Design review of the part built by this model. Coordinates are the model's own, in mm. A direction names the side the tool comes from. Give positions to 0.01 mm unless a question says otherwise; leave off trailing zeros. Write each loop counter-clockwise with the first axis right and the second up, starting at its lowest first coordinate (ties: lowest second). Pieces come first, ordered by that corner, then holes. Notation, with made-up numbers: M -39,69.25 L -32,69.25 A24 cw -32,85.25 Z; hole C 59,-37 d4. An arc over 180 degrees is marked long. One line per item, written item: value. Start each with the question number.
```python
from build123d import *

# Parameters (mm, degrees)
SKETCH1_W           = 80
SKETCH1_H           = 4
SKETCH1_W_2         = 10
BOSS_EXTRUDE1_DEPTH = 20
CUT_EXTRUDE2_REACH  = 92
SKETCH2_R           = 2.7
CUT_EXTRUDE3_REACH  = 14
SKETCH4_R           = 1.7
SKETCH5_R           = 3.7
SKETCH5_R_2         = 1.7
BOSS_EXTRUDE2_DEPTH = 3
SKETCH6_R           = 4.3
CUT_EXTRUDE4_DEPTH  = 5
CUT_EXTRUDE5_DEPTH  = 3


with BuildPart() as part:
    # Sketch1 → Boss-Extrude1 (new body)
    with BuildSketch(Plane(origin=(0, 0, 0), x_dir=(1, 0, 0), z_dir=(0, 1, 0))):
        with Locations((40, -2)):
            Rectangle(SKETCH1_W, SKETCH1_H)
        Polygon((80, 8), (80, 0), (80, -4), (80, -40.5), (90, -40.5), (90, -36.5), (90, 4), (90, 8), align=None)
        with Locations((95, 6)):
            Rectangle(SKETCH1_W_2, SKETCH1_H)
        with Locations((95, -38.5)):
            Rectangle(SKETCH1_W_2, SKETCH1_H)
    extrude(amount=BOSS_EXTRUDE1_DEPTH)

    # Sketch2 → Cut-Extrude2 (cut, up to next)
    with BuildSketch(Plane(origin=(90, 0, 0), x_dir=(0, 0, -1), z_dir=(1, 0, 0)), mode=Mode.PRIVATE) as cut_extrude2_sk1:
        with Locations((-16.25, 10)):
            Circle(SKETCH2_R)
    cut_extrude2_tool1 = extrude(cut_extrude2_sk1.sketch, amount=-CUT_EXTRUDE2_REACH, mode=Mode.PRIVATE) & part.part
    add(cut_extrude2_tool1.solids().sort_by_distance((90, 10, 16.25))[0], mode=Mode.SUBTRACT)

    # Sketch4 → Cut-Extrude3 (cut, up to next)
    with BuildSketch(Plane.XY.offset(4), mode=Mode.PRIVATE) as cut_extrude3_sk1:
        with Locations((16.48, 10)):
            Circle(SKETCH4_R)
    cut_extrude3_tool1 = extrude(cut_extrude3_sk1.sketch, amount=-CUT_EXTRUDE3_REACH, mode=Mode.PRIVATE) & part.part
    add(cut_extrude3_tool1.solids().sort_by_distance((16.48, 10, 4))[0], mode=Mode.SUBTRACT)
    # Sketch4 → Cut-Extrude3 (cut, up to next)
    with BuildSketch(Plane.XY.offset(4), mode=Mode.PRIVATE) as cut_extrude3_sk2:
        with Locations((63.52, 10)):
            Circle(SKETCH4_R)
    cut_extrude3_tool2 = extrude(cut_extrude3_sk2.sketch, amount=-CUT_EXTRUDE3_REACH, mode=Mode.PRIVATE) & part.part
    add(cut_extrude3_tool2.solids().sort_by_distance((63.52, 10, 4))[0], mode=Mode.SUBTRACT)

    # Sketch5 → Boss-Extrude2 (add)
    with BuildSketch(Plane.XY.offset(4)):
        with Locations((16.48, 10)):
            Circle(SKETCH5_R)
        with Locations((16.48, 10)):
            Circle(SKETCH5_R_2, mode=Mode.SUBTRACT)
        with Locations((63.52, 10)):
            Circle(SKETCH5_R)
        with Locations((63.52, 10)):
            Circle(SKETCH5_R_2, mode=Mode.SUBTRACT)
    extrude(amount=BOSS_EXTRUDE2_DEPTH)

    # Sketch6 → Cut-Extrude4 (cut)
    with BuildSketch(Plane.ZY.offset(-80)):
        with Locations((16.25, 10)):
            Circle(SKETCH6_R)
    extrude(amount=-CUT_EXTRUDE4_DEPTH, mode=Mode.SUBTRACT)

    # Sketch7 → Cut-Extrude5 (cut)
    with BuildSketch(Plane(origin=(0, 0, 0), x_dir=(-1, 0, 0), z_dir=(0, 0, -1))):
        Polygon((-60.77, 8.41228676), (-60.77, 11.58771324), (-63.52, 13.175426481), (-66.27, 11.58771324), (-66.27, 8.41228676), (-63.52, 6.824573519), align=None)
        Polygon((-13.73, 8.41228676), (-13.73, 11.58771324), (-16.48, 13.175426481), (-19.23, 11.58771324), (-19.23, 8.41228676), (-16.48, 6.824573519), align=None)
    extrude(amount=-CUT_EXTRUDE5_DEPTH, mode=Mode.SUBTRACT)


solid = part.part
```
Q1. Take a section at A-A, the plane z = 16.25. Give the boundary of the cut face in (x, y).
Q2. Machinability: for faces 1 (the face through (82.46, 11.29, 20.35)), 2 (the face through (39, 10, 0)), 3 (the face through (15.12, 7.61, 1.48)), which of the approach directions +Z, -Z, +X, -X, +Y, -Y give a long, thin tool a straight path to every point of the face, cutting with its end or side? Answer none if there is none.
Q3. For P1, Ø2.5, axis at y = 9.5, z = 1, coming from the +X side; P2, Ø6, axis at x = 62.5, y = 10, coming from the -Z side; P3, Ø4.5, axis at x = 63.52, y = 10, coming from the -Z side, all flat-tipped, find the tip position at first contact; note any pin that passes through.
Q4. Take a section at B-B, the plane y = 10. State how many separate pieces and enclosed holes the cut face has, then the cut area to 3 significant figures.
Q5. Take a section at C-C, the plane x = 77.5. Give the boundary of the cut face in (y, z), then the cut area to 3 significant figures.
Q6. The part is to be moulded in two halves that separate along Y. For faces 4 (the face through (0, 10, 2)), 5 (the face through (66.938, 8.583, 5.479)), 6 (the face through (13.73, 10, 1)), 7 (the face through (64.88, 12.39, 1.48)), say which applies: pulls with the +Y half, pulls with the -Y half, needs draft (parallel to the pull), parting line crosses it, or undercut.
Q7. Take a section at D-D, the plane z = 25. Give the boundary of the cut face in (x, y), then the cut area to 3 significant figures.
Q8. Wall thickness on line 1 (Y direction, x = 16.48, z = 3.2); line 2 (Y direction, x = 86, z = 16); line 3 (X direction, y = 6, z = 11.5): over which ranges is each line inside the solid? List them lowest first. Write a range as from..to.
Results list:
1. outline: M 80,0 L 90,0 L 90,7.3 L 85,7.3 L 85,5.7 L 80,5.7 Z; M 80,14.3 L 85,14.3 L 85,12.7 L 90,12.7 L 90,20 L 80,20 Z
2. face 1: -X
2. face 2: -Z, -X, +Y, -Y
2. face 3: -Z
3. P1: stops at x = 90
3. P2: stops at z = 0
3. P3: stops at z = 3
4. separate pieces: 4
4. enclosed holes: 0
4. area: 799 mm^2
5. outline: M 0,0 L 20,0 L 20,4 L 0,4 Z
5. area: 80.0 mm^2
6. face 4: needs draft
6. face 5: parting line crosses it
6. face 6: undercut
6. face 7: undercut
7. outline: M 80,0 L 90,0 L 90,20 L 80,20 Z
7. area: 200 mm^2
8. line 1: y = 0..8.3, 11.7..20
8. line 2: y = 0..7.31, 12.69..20
8. line 3: x = 80..90
